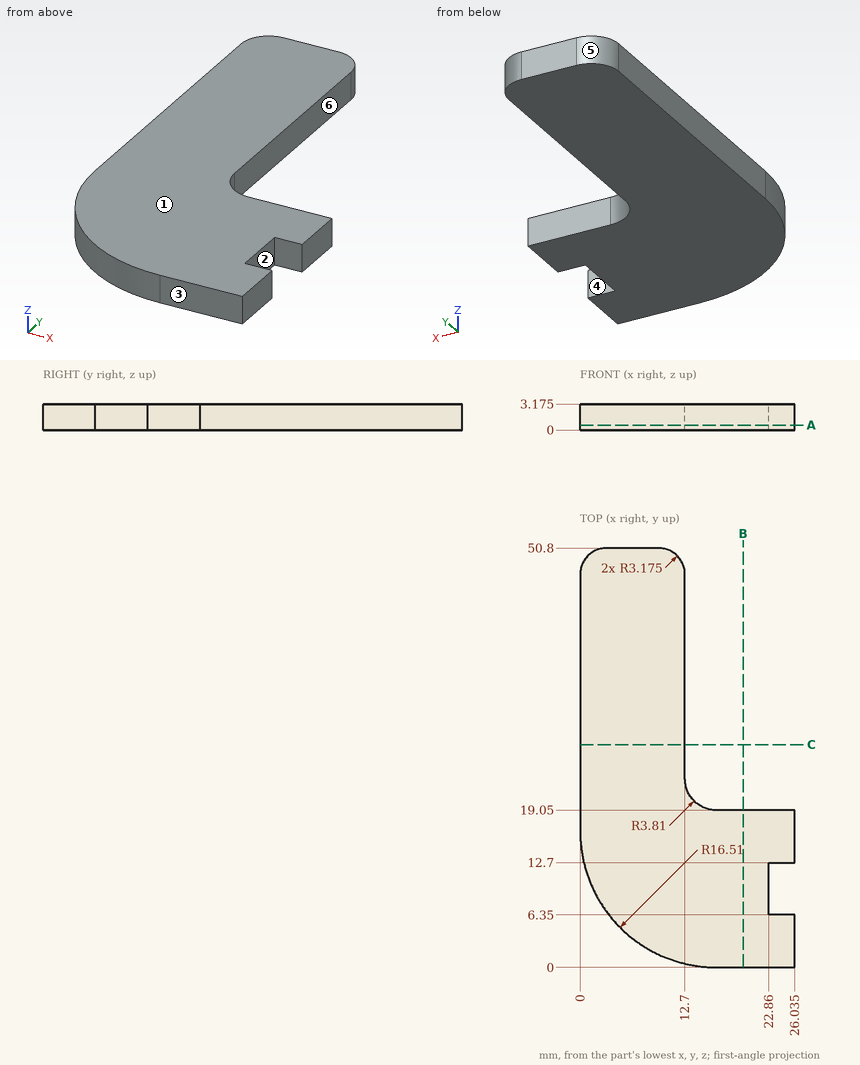
The drawing under review shows one solid part. Ordinate dimensions are in mm from its lowest x, y, z. A direction names the side the tool comes from. Round coordinates to 2 decimals unless told otherwise and drop trailing zeros. Order: outer loops, then holes, each group sorted by start corner. A loop starts at its lowest first (then second) coordinate and runs counter-clockwise, first axis right, second up. Notation, with made-up numbers: (-1.5, -22) -> (24.5, -22) arc R19 cw to (24.5, -8) -> close; hole circle Ø10 at (45.5, -37.5). An arc over 180 degrees is marked (long way). Use a Markdown table: item, result.
Q1. We need section B-B on x = 19.75. Write out the cut boundary in (y, z) (3 decimals), then the cut area to 3 significant figures.
Values:
| item | result |
|---|---|
| outline | (0, 0) -> (19.05, 0) -> (19.05, 3.175) -> (0, 3.175) -> close |
| area | 60.5 mm^2 |
Q2. We need section A-A on z = 0.6. Write out the cut boundary in (x, y) (3 decimals).
Values:
| item | result |
|---|---|
| outline | (0, 16.51) arc R16.51 ccw to (16.51, 0) -> (26.035, 0) -> (26.035, 6.35) -> (22.86, 6.35) -> (22.86, 12.7) -> (26.035, 12.7) -> (26.035, 19.05) -> (16.51, 19.05) arc R3.81 cw to (12.7, 22.86) -> (12.7, 47.625) arc R3.175 ccw to (9.525, 50.8) -> (3.175, 50.8) arc R3.175 ccw to (0, 47.625) -> close |
Q3. Tool access review of the marked faces 4, 5 and 6: name each direction out of +Z, -Z, +X, -X, +Y, -Y from which nothing blocks a thin tool from reaching the whole face with its end or side.
Values:
| item | result |
|---|---|
| face 4 | +Z, -Z, +X |
| face 5 | +Z, -Z, -X, +Y |
| face 6 | +Z, -Z, +X, +Y |
Q4. For line 1 (Y direction, x = 18.25, z = 2.9); line 2 (X direction, y = 28, z = 0.85); line 3 (X direction, y = 7.5, z = 2.2), list the stretches that pass through material, from the lowest coordinate up.
Values:
| item | result |
|---|---|
| line 1 | y = 0 to 19.05 |
| line 2 | x = 0 to 12.7 |
| line 3 | x = 2.68 to 22.86 |
Q5. We need section C-C on y = 27. Write out the cut boundary in (x, z) (3 decimals), then the cut area to 3 significant figures.
Values:
| item | result |
|---|---|
| outline | (0, 0) -> (12.7, 0) -> (12.7, 3.175) -> (0, 3.175) -> close |
| area | 40.3 mm^2 |
Q6. Clearance check with flat-ended pins moving along their axes: P1, Ø1, axis at x = 6, z = 0.5, coming from the -Y side; P2, Ø1.6, axis at y = 33, z = 1, coming from the +X side; P3, Ø1, axis at x = 20.5, z = 2, coming from the +Y side. State where each tip first meets the part, or that it passes through.
Values:
| item | result |
|---|---|
| P1 | stops at y = 3.38 |
| P2 | stops at x = 12.7 |
| P3 | stops at y = 19.05 |
Q7. Mouldability with a two-part tool opening along Y and no side actions: class the marked faces 1, 2 and 3 as +Y half, -Y half, draft (parallel to the pull), parting line (faces both ways), or undercut.
Values:
| item | result |
|---|---|
| face 1 | draft |
| face 2 | undercut |
| face 3 | -Y half |
